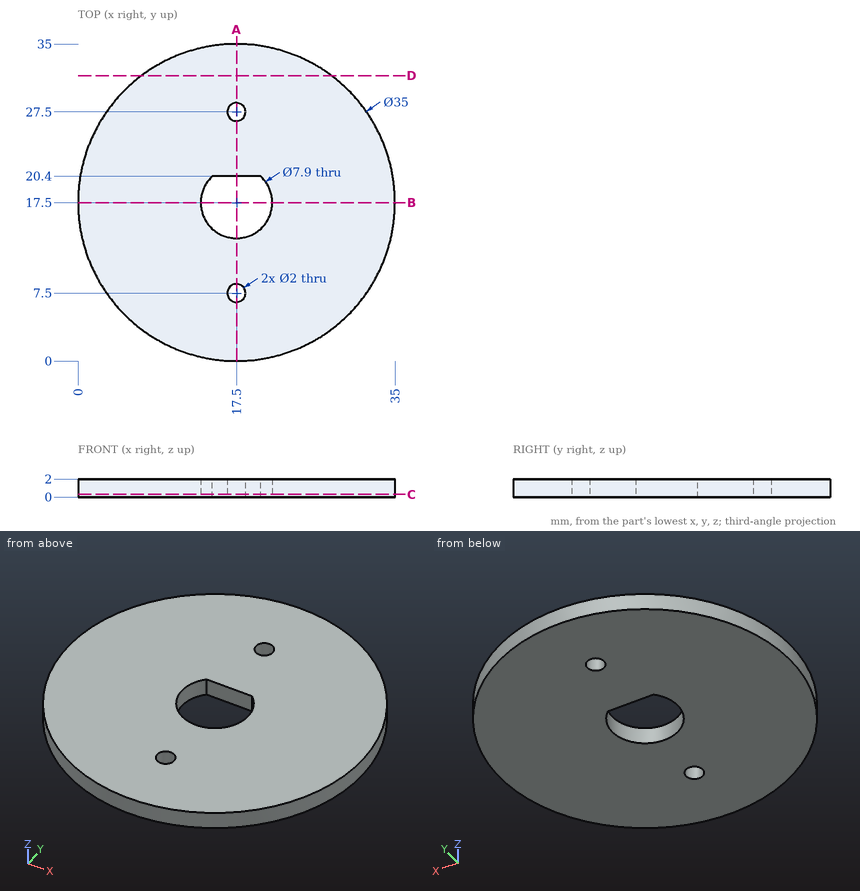
The figure shows three views and two pictorial views of one solid part (mm, origin at its lowest corner). Answer the questions. Coordinates: 2 decimals unless noted, no trailing zeros. Order: outer loops, then holes, each group sorted by start corner. A loop starts at its lowest first (then second) coordinate and runs counter-clockwise, first axis right, second up. Notation, with made-up numbers: (36, 6.5) - (48, 6.5) arc R21 cw to (48, 34.5) - close; hole circle Ø8 at (81, -1.5). An arc over 180 degrees is marked (long way). Answer as a JSON object with one key per item and string values.
1. Find section D-D on y = 31.5. Determine the outline of the cut face in (x, z).
Output values:
{"outline": "(7, 0) - (28, 0) - (28, 2) - (7, 2) - close"}
2. This flat-tipped pin is pushed along its axis until it touches: P1, Ø0.6, axis at x = 18.5, z = 1, coming from the -Y side. Where does it stop, or does it pass through?
Output values:
{"P1": "stops at y = 0.01"}
3. Find section A-A on x = 17.5. Determine the outline of the cut face in (y, z), plus the area to 3 significant figures.
Output values:
{"outline": "(0, 0) - (6.5, 0) - (6.5, 2) - (0, 2) - close; (8.5, 0) - (13.55, 0) - (13.55, 2) - (8.5, 2) - close; (20.4, 0) - (26.5, 0) - (26.5, 2) - (20.4, 2) - close; (28.5, 0) - (35, 0) - (35, 2) - (28.5, 2) - close", "area": "48.3 mm²"}
4. Find section B-B on y = 17.5. Determine the outline of the cut face in (x, z), plus the area to 3 significant figures.
Output values:
{"outline": "(0, 0) - (13.55, 0) - (13.55, 2) - (0, 2) - close; (21.45, 0) - (35, 0) - (35, 2) - (21.45, 2) - close", "area": "54.2 mm²"}
5. Find section C-C on z = 0.3. Determine the outline of the cut face in (x, y), plus the area to 3 significant figures.
Output values:
{"outline": "circle Ø35 at (17.5, 17.5); hole (14.82, 20.4) arc R3.95 ccw (long way) to (20.18, 20.4) - close; hole circle Ø2 at (17.5, 7.5); hole circle Ø2 at (17.5, 27.5)", "area": "911 mm²"}
6. Consider line 1 (X direction, y = 18, z = 0.9); line 2 (Y direction, x = 15.5, z = 0.9); line 3 (Y direction, x = 19, z = 1.6). Determine where each line is inside the solid, lowest interval first.
Output values:
{"line 1": "x = 0.01 to 13.58, 21.42 to 34.99", "line 2": "y = 0.11 to 14.09, 20.4 to 34.89", "line 3": "y = 0.06 to 13.85, 20.4 to 34.94"}
